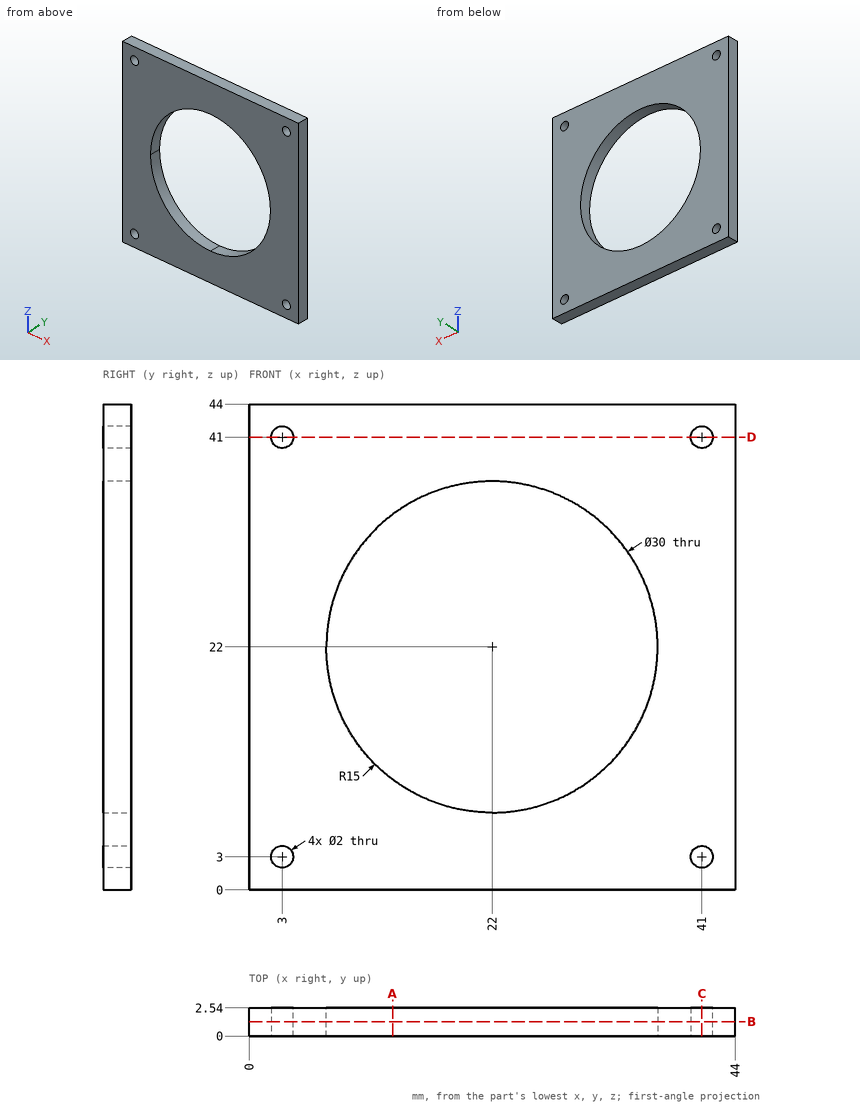
Here's the drawing with two shaded views (mm, measured from the low corner). I have some questions. Coordinates: 2 decimals unless noted, no trailing zeros. Write each loop counter-clockwise with the first axis right and the second up, starting at its lowest first coordinate (ties: lowest second). Pieces come first, ordered by that corner, then holes. Notation, with made-up numbers: M 32,-5.5 L 57,-5.5 A16 cw 57,16.5 Z; hole C -39,-4.75 d4. An arc over 180 degrees is marked long. Write item = value, one per line. Start each with the question number.
Q1. I'm going to push a flat-ended pin straight in: pin 1 (3 mm diameter, centred on x = 3, z = 3, fed in from +Y). Where does the tip first touch, or does it pass through?
Q2. If we section it at B-B, the plane y = 1.3: Write out the boundary of the cut face in (x, z), then the cut area to 3 significant figures.
Q3. If we section it at D-D, the plane z = 41: Write out the boundary of the cut face in (x, y).
Q4. If we section it at A-A, the plane x = 13: Write out the boundary of the cut face in (y, z).
Q5. If we section it at C-C, the plane x = 41: Write out the boundary of the cut face in (y, z).
Q6. If I drill on L1, parallel to Z at x = 41, y = 1.5; L2, parallel to Z at x = 22, y = 1.4, over which ranges is the centre line in solid material (lowest first)? Write a range as [from, to].
Check sheet entries:
q1.pin_1 = 2.54
q2.outline = M 0,0 L 44,0 L 44,44 L 0,44 Z; hole C 3,3 d2; hole C 3,41 d2; hole C 22,22 d30; hole C 41,3 d2; hole C 41,41 d2
q2.area = 1,220 mm²
q3.outline = M 0,0 L 2,0 L 2,2.54 L 0,2.54 Z; M 4,0 L 40,0 L 40,2.54 L 4,2.54 Z; M 42,0 L 44,0 L 44,2.54 L 42,2.54 Z
q4.outline = M 0,0 L 2.54,0 L 2.54,10 L 0,10 Z; M 0,34 L 2.54,34 L 2.54,44 L 0,44 Z
q5.outline = M 0,0 L 2.54,0 L 2.54,2 L 0,2 Z; M 0,4 L 2.54,4 L 2.54,40 L 0,40 Z; M 0,42 L 2.54,42 L 2.54,44 L 0,44 Z
q6.L1 = [0, 2], [4, 40], [42, 44]
q6.L2 = [0, 7], [37, 44]
